Autodesk Inventor part; units mm, degrees
ref_plane "YZ Plane" through (0, 0, 0) normal (1, 0, 0) x (0, 1, 0)
ref_plane "XZ Plane" through (0, 0, 0) normal (0, 1, 0) x (-1, 0, 0)
ref_plane "XY Plane" through (0, 0, 0) normal (0, 0, 1) x (1, 0, 0)
sketch "Sketch1" plane through (0, 0, 0) normal (0, 1, 0) x (-1, 0, 0)
  line L0 (95.25, 50.8) -> (-95.25, 50.8)
  line L1 (-95.25, 50.8) -> (-95.25, -50.8)
  line L2 (-95.25, -50.8) -> (95.25, -50.8)
  line L3 (95.25, -50.8) -> (95.25, 50.8)
  line L4 (95.25, 50.8) -> (-95.25, -50.8) construction
  line L5 (-95.25, 50.8) -> (95.25, -50.8) construction
  circle A0 centre (82.55, -38.1) radius 3.302
  circle A1 centre (-82.55, -38.1) radius 3.302
  circle A2 centre (-82.7024, 38.1) radius 3.302
  circle A3 centre (82.55, 38.1) radius 3.302
  line L6 (40.9111, -12.7) -> (-47.9889, -12.7) construction
  line L7 (40.9111, 12.7) -> (-47.9889, 12.7) construction
  circle A4 centre (23.8125, -12.7) radius 2.413
  circle A5 centre (-23.8125, -12.7) radius 2.413
  circle A6 centre (23.8125, 12.7) radius 2.413
  circle A7 centre (-23.8125, 12.7) radius 2.413
  point P0 (0, 0)
  dimension "d0" = 190.5
  dimension "d1" = 101.6
  dimension "d2" = 6.604
  dimension "d3" = 12.7
  dimension "d4" = 12.7
  dimension "d5" = 6.604
  dimension "d6" = 12.7
  dimension "d7" = 6.604
  dimension "d8" = 12.7
  dimension "d9" = 6.604
  dimension "d10" = 88.9
  dimension "d11" = 88.9
  dimension "d12" = 25.4
  dimension "d13" = 12.7
  dimension "d14" = 4.826
  dimension "d15" = 4.826
  dimension "d16" = 47.625
  dimension "d17" = 23.8125
  dimension "d18" = 4.826
  dimension "d19" = 4.826
  dimension "d22" = 12.7
  dimension "d23" = 12.7
extrude "Extrusion1" add sketch "Sketch1" along normal blind 6.35
properties part number "SequenceMachine_ManifoldPlate"
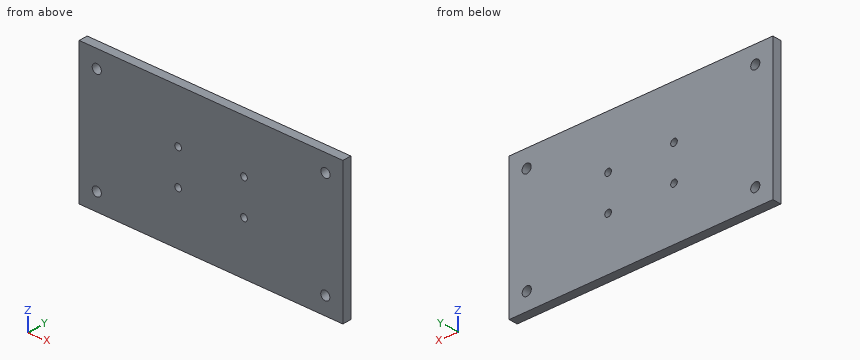
For this review, take the finished solid that the model builds, in its own axes (mm). Coordinates: 2 decimals unless noted, no trailing zeros. Write each loop counter-clockwise with the first axis right and the second up, starting at its lowest first coordinate (ties: lowest second). Pieces come first, ordered by that corner, then holes. Notation, with made-up numbers: (36, 18) -> (92, 18) arc R25 cw to (92, 41) -> close; hole circle Ø7 at (-17.5, 76.25). An arc over 180 degrees is marked (long way). Write each question's results on one line, items separated by ' | '. Start each with the question number.
1) Consider section A-A (z = 12.7). Write out the cut boundary in (x, y), plus the area to 3 significant figures.
2) Wall thickness on L1, parallel to Z at x = 82.55, y = 4.5; L2, parallel to Z at x = -81, y = 2.5; L3, parallel to X at y = 2.75, z = 38: over which ranges is each line inside the solid? List them lowest first. Write a range as [from, to].
3) Consider section B-B (x = -82.55). Write out the cut boundary in (y, z).
4) Insertion check: pin 1 (4.5 mm diameter, centred on x = -23.81, z = -12.7, fed in from +Y). The pin has a flat end and moves straight along its axis. Give the tip position at first contact, or say it passes through.
Geometry says:
1) outline: (-95.25, 0) -> (-26.23, 0) -> (-26.23, 6.35) -> (-95.25, 6.35) -> close; (-21.4, 0) -> (21.4, 0) -> (21.4, 6.35) -> (-21.4, 6.35) -> close; (26.23, 0) -> (95.25, 0) -> (95.25, 6.35) -> (26.23, 6.35) -> close | area: 1,150 mm^2
2) L1: [-50.8, -41.4], [-34.8, 34.8], [41.4, 50.8] | L2: [-50.8, -41.02], [-35.18, 35.18], [41.02, 50.8] | L3: [-95.25, -85.85], [-79.25, 79.4], [86, 95.25]
3) outline: (0, -50.8) -> (6.35, -50.8) -> (6.35, -41.4) -> (0, -41.4) -> close; (0, -34.8) -> (6.35, -34.8) -> (6.35, 34.8) -> (0, 34.8) -> close; (0, 41.4) -> (6.35, 41.4) -> (6.35, 50.8) -> (0, 50.8) -> close
4) pin 1: through
